Geometry: final body of the model. Coordinates: model frame, mm. Face numbers are marked on the shaded views. A direction names the side the tool comes from. Coordinates: 2 decimals unless noted, no trailing zeros. Order: outer loops, then holes, each group sorted by start corner. A loop starts at its lowest first (then second) coordinate and runs counter-clockwise, first axis right, second up. Notation, with made-up numbers: M -8,-4.5 L -3,-4.5 A7 cw -3,7.5 Z; hole C 67.25,19 d1. An arc over 180 degrees is marked long. Use CSV: the item, a comma, the result in double quotes. Start each with the question number.
Q1. Section query C-C, the plane z = -19.5. Output: boundary loops of the cut face in (x, y).
Q2. First-contact query: P1, Ø4, axis at x = 2.5, z = -15, coming from the +Y side (3 decimals); P2, Ø5, axis at x = 0.5, y = 6.5, coming from the +Z side; P3, Ø3, axis at x = -1.5, z = 35.5, coming from the +Y side (3 decimals). Flat tips, straight axial feed; report the tip coordinate or a pass-through.
Q3. Access query for the marked faces 1 and 2. Directions: +Z, -Z, +X, -X, +Y, -Y. A direction counts if a zero-diameter tool reaches every point of the face in a straight line with its end or side. Return the directions, or none.
Q4. Section query A-A, the plane x = 0. State how many separate pieces and enclosed holes the cut face has, and give its area (3 significant figures).
Q5. Mould query, pull axis Z, two halves, no side actions, for the marked faces 3 and 4. Classes: +Z half, -Z half, draft (parallel to the pull), parting line (faces both ways), or undercut.
Q6. Section query B-B, the plane z = -32.5. Output: boundary loops of the cut face in (x, y) (3 decimals).
Q7. Ray query, probe 1 along Y at (x, z) = (0, -42); probe 2 along Z at (x, y) = (0.75, 8); probe 3 along Y at (x, z) = (-0.5, 3) (3 decimals). Return the intervals inside material, ascending.
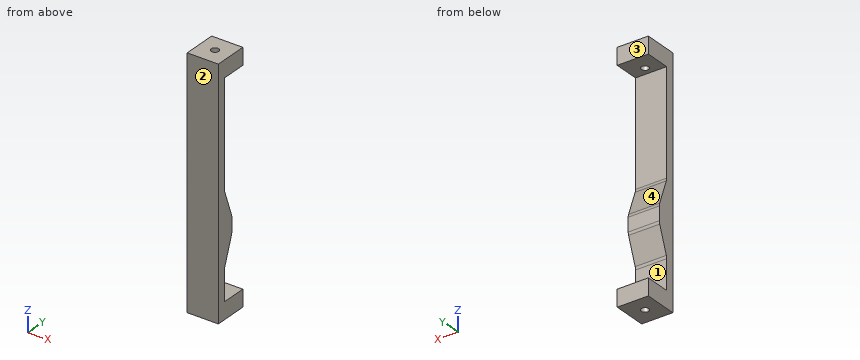
from build123d import *

# Parameters (mm, degrees)
SKETCH1_W           = 11.7475
SKETCH1_H           = 91.567
BOSS_EXTRUDE1_DEPTH = 3.175
SKETCH5_W           = 11.7475
SKETCH5_H           = 9.525
BOSS_EXTRUDE2_DEPTH = 6.35
SKETCH4_R           = 1.399999994
CUT_EXTRUDE1_DEPTH  = 92.567
BOSS_EXTRUDE3_DEPTH = 11.7475
FILLET1_R           = 3.175


with BuildPart() as part:
    # Sketch1 → Boss-Extrude1 (new body)
    with BuildSketch(Plane(origin=(0, 0, 0), x_dir=(1, 0, 0), z_dir=(0, 1, 0))):
        Rectangle(SKETCH1_W, SKETCH1_H)
    extrude(amount=BOSS_EXTRUDE1_DEPTH)

    # Sketch5 → Boss-Extrude2 (add)
    with BuildSketch(Plane.XY.offset(45.7835)):
        with Locations((0, 7.9375)):
            Rectangle(SKETCH5_W, SKETCH5_H)
    boss_extrude2 = extrude(amount=-BOSS_EXTRUDE2_DEPTH)

    # Mirror1: Boss-Extrude2 across plane
    add(boss_extrude2.mirror(Plane.XY))

    # Sketch4 → Cut-Extrude1 (cut, through all)
    with BuildSketch(Plane.XY.offset(45.7835)):
        with Locations((0, 6.35)):
            Circle(SKETCH4_R)
    extrude(amount=-CUT_EXTRUDE1_DEPTH, mode=Mode.SUBTRACT)

    # Sketch6 → Boss-Extrude3 (add)
    with BuildSketch(Plane.ZY.offset(5.87375)):
        Polygon((-17.2085, 6.985), (-10.8585, 6.985), (-0.390611032, 3.175), (-27.676388968, 3.175), align=None)
    extrude(amount=-BOSS_EXTRUDE3_DEPTH)

    # Fillet1
    fillet1_edges = [part.edges().sort_by_distance(p)[0] for p in [
        (0, 3.175, -27.676388968),
        (0, 6.985, -17.2085),
        (0, 6.985, -10.8585),
        (0, 3.175, -0.390611032),
    ]]
    fillet(fillet1_edges, radius=FILLET1_R)


solid = part.part
Responses:
1,outline,"M -5.87,0 L 5.87,0 L 5.87,6.15 L -5.87,6.15 Z"
2,P1,"stops at y = 6.985"
2,P2,"stops at z = 45.78"
2,P3,"stops at y = 3.175"
3,face 1,"+X, -X, +Y"
3,face 2,"+Z, -Z, +X, -X, -Y"
4,separate pieces,"3"
4,enclosed holes,"0"
4,area,"440 mm²"
5,face 3,"draft"
5,face 4,"undercut"
6,outline,"M -5.874,0 L 5.874,0 L 5.874,3.175 L -5.874,3.175 Z"
7,probe 1,"y = 0 to 4.95, 7.75 to 12.7"
7,probe 2,"z = -45.78 to -39.43, 39.43 to 45.78"
7,probe 3,"y = 0 to 3.175"
